Answer from the drawing. Dimensions are ordinates in mm from the lowest x, y and z of the part. A direction names the side the tool comes from. Round coordinates to 2 decimals unless told otherwise and drop trailing zeros. Loops run counter-clockwise (first coordinate to the right, second up) from the corner with the lowest first, then second, coordinate; pieces in that order, holes last. Notation, with made-up numbers: (2, 71) - (54, 71) arc R14 cw to (54, 81) - close; hole circle Ø11 at (3, -7.5). An arc over 180 degrees is marked (long way). One line per question, with ' | ' between items. Start each with the question number.
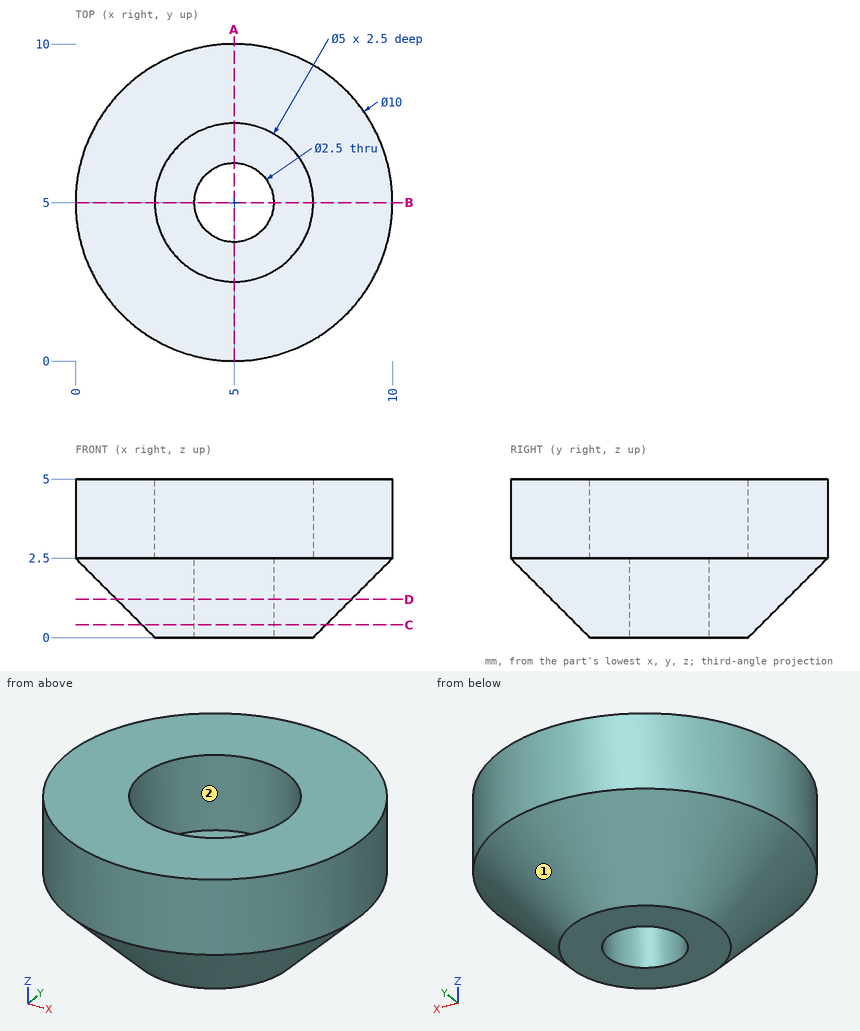
(1) Find section D-D on z = 1.2. Write down the section's boundary in (x, y).
(2) A tool of negligible diameter and unlimited length cuts with its end or side. For the marked faces 1 and 2, from which of +Z, -Z, +X, -X, +Y, -Y can it reach the whole face along a straight path? Write none if from no direction.
(3) Find section A-A on x = 5. Write down the section's boundary in (y, z).
(4) Find section C-C on z = 0.4. Write down the section's boundary in (x, y), plus the area to 3 significant figures.
(5) Consider L1, parallel to Y at x = 5, z = 3.95; L2, parallel to X at y = 6, z = 0.25; L3, parallel to Y at x = 6.75, z = 4.15. Determine where each line is inside the solid, lowest interval first.
(6) Each of these flat-tipped pins is pushed along its axis until it touches: P1, Ø1, axis at y = 6, z = 3, coming from the -X side; P2, Ø1.5, axis at x = 6.5, y = 2, coming from the -Z side; P3, Ø1.5, axis at x = 4, z = 2.5, coming from the -Y side. Where does it stop, or does it pass through?
Answer below:
1) outline: circle Ø7.4 at (5, 5); hole circle Ø2.5 at (5, 5)
2) face 1: -Z | face 2: +Z
3) outline: (0, 2.5) - (2.5, 0) - (3.75, 0) - (3.75, 2.5) - (2.5, 2.5) - (2.5, 5) - (0, 5) - close; (6.25, 0) - (7.5, 0) - (10, 2.5) - (10, 5) - (7.5, 5) - (7.5, 2.5) - (6.25, 2.5) - close
4) outline: circle Ø5.8 at (5, 5); hole circle Ø2.5 at (5, 5) | area: 21.5 mm2
5) L1: 0 to 2.5, 7.5 to 10 | L2: 2.44 to 4.25, 5.75 to 7.56 | L3: 0.32 to 3.21, 6.79 to 9.68
6) P1: x = 0.03 | P2: z = 0.1 | P3: y = 0.01
